```python
from build123d import *

# Parameters (mm, degrees)
ESBO_O1_R                = 6.35
RESSALTO_EXTRUS_O1_DEPTH = 160
ESBO_O2_OUTSIDE_W        = 46.9
ESBO_O2_OUTSIDE_H        = 46.9
ESBO_O2_OUTSIDE_R        = 5
CORTE_EXTRUS_O1_DEPTH    = 12
ESBO_O4_OUTSIDE_W        = 46.9
ESBO_O4_OUTSIDE_H        = 46.9
ESBO_O4_OUTSIDE_R        = 3.5
CORTE_EXTRUS_O2_DEPTH    = 3.6
FILETE1_R                = 0.2
CHANFRO2_SIZE            = 2
CHANFRO2_SIZE2           = 3.464101615
CHANFRO3_SIZE            = 1.5
CHANFRO3_SIZE2           = 2.598076211


with BuildPart() as part:
    # Esboço1 → Ressalto-extrusão1 (new body)
    with BuildSketch(Plane.XY):
        Circle(ESBO_O1_R)
    extrude(amount=RESSALTO_EXTRUS_O1_DEPTH)

    # Esboço2 outside → Corte-extrusão1 (cut)
    with BuildSketch(Plane(origin=(0, 0, 0), x_dir=(-1, 0, 0), z_dir=(0, 0, -1))):
        Rectangle(ESBO_O2_OUTSIDE_W, ESBO_O2_OUTSIDE_H)
        Circle(ESBO_O2_OUTSIDE_R, mode=Mode.SUBTRACT)
    extrude(amount=-CORTE_EXTRUS_O1_DEPTH, mode=Mode.SUBTRACT)

    # Esboço4 outside → Corte-extrusão2 (cut)
    with BuildSketch(Plane(origin=(0, 0, 12), x_dir=(-1, 0, 0), z_dir=(0, 0, -1))):
        Rectangle(ESBO_O4_OUTSIDE_W, ESBO_O4_OUTSIDE_H)
        Circle(ESBO_O4_OUTSIDE_R, mode=Mode.SUBTRACT)
    extrude(amount=CORTE_EXTRUS_O2_DEPTH, mode=Mode.SUBTRACT)

    # Filete1
    filete1_edges = [part.edges().sort_by_distance(p)[0] for p in [
        (5, 0, 8.4),
    ]]
    fillet(filete1_edges, radius=FILETE1_R)

    # Chanfro2
    chanfro2_edges = [part.edges().sort_by_distance(p)[0] for p in [
        (5, 0, 0),
    ]]
    chanfro2_side = [part.faces().sort_by_distance(p)[0] for p in [
        (5, 0, 4.1),
    ]]
    chamfer(chanfro2_edges, length=CHANFRO2_SIZE, length2=CHANFRO2_SIZE2, reference=chanfro2_side[0])

    # Chanfro3
    chanfro3_edges = [part.edges().sort_by_distance(p)[0] for p in [
        (-6.35, 0, 12),
    ]]
    chanfro3_side = [part.faces().sort_by_distance(p)[0] for p in [
        (-6.35, 0, 86),
    ]]
    chamfer(chanfro3_edges, length=CHANFRO3_SIZE, length2=CHANFRO3_SIZE2, reference=chanfro3_side[0])


solid = part.part
```
The listing builds one solid part. Answer for the finished solid, in the listing's coordinates (mm). A direction names the side the tool comes from. Round coordinates to 2 decimals unless told otherwise and drop trailing zeros. Loops run counter-clockwise (first coordinate to the right, second up) from the corner with the lowest first, then second, coordinate; pieces in that order, holes last.
Q1. For a pull along Z with two mould halves and no side action, classify faces 3 (the face through (1.08, -4.88, 5.06)), 4 (the face through (-3.233, -1.341, 10.225)), 5 (the face through (0, 0, 160)) as released by +Z, released by -Z, zero draft, split by the parting line, or undercut.
Q2. Given pin 1 Ø2 at (x, z) = (-2.5, 34.5) entering from +Y; pin 2 Ø2 at (y, z) = (4, 45) entering from +X; pin 3 Ø2 at (x, y) = (-1.5, -4.5) entering from -Z, each flat-ended and moving along its own axis, determine where each tip first touches the part or whether it passes through.
Q3. Find the intervals of material crossed by line 1 (Y direction, x = -0.5, z = 149.5); line 2 (X direction, y = -0.25, z = 52.5); line 3 (Z direction, x = 3.5, y = 3.5), in increasing order.
Q4. Section C-C, the plane z = 63 is taken. Determine the outline of the cut face in (x, y).
Q5. Section A-A, the plane x = 0 is taken. Determine the outline of the cut face in (y, z).
Q6. Which of the six approach directions +Z, -Z, +X, -X, +Y, -Y give full straight-line access (tool end or side, diameter ignored) to faces 1 (the face through (0, -4, 8.4)), 2 (the face through (-1.38, -6.2, 85.72))?
Completed:
1. face 3: zero draft
1. face 4: undercut
1. face 5: released by +Z
2. pin 1: stops at y = 6.17
2. pin 2: stops at x = 5.6
2. pin 3: stops at z = 1.27
3. line 1: y = -6.33 to 6.33
3. line 2: x = -6.35 to 6.35
3. line 3: z = 1.97 to 8.33, 12.69 to 160
4. outline: circle Ø12.7 at (0, 0)
5. outline: (-6.35, 13.5) - (-3.75, 12) - (-3.5, 12) - (-3.5, 8.4) - (-4.8, 8.4) arc R0.2 ccw to (-5, 8.2) - (-5, 2) - (-1.54, 0) - (1.54, 0) - (5, 2) - (5, 8.2) arc R0.2 ccw to (4.8, 8.4) - (3.5, 8.4) - (3.5, 12) - (3.75, 12) - (6.35, 13.5) - (6.35, 160) - (-6.35, 160) - close
6. face 1: none
6. face 2: +Z, -Z
